```python
from build123d import *

# Parameters (mm, degrees)
SKETCH_W     = 50
SKETCH_H     = 50
PAD_DEPTH    = 3
SKETCH001_R  = 1.05
POCKET_DEPTH = 3.001
CHAMFER_SIZE = 1


with BuildPart() as part:
    # Sketch → Pad (new body)
    with BuildSketch(Plane.XY):
        Rectangle(SKETCH_W, SKETCH_H)
    extrude(amount=PAD_DEPTH)

    # Sketch001 (on Face6 of Pad) → Pocket (cut, through all)
    with BuildSketch(Plane.XY.offset(3)):
        with Locations((-17, 17)):
            Circle(SKETCH001_R)
        with Locations((17, 17)):
            Circle(SKETCH001_R)
        with Locations((17, -17)):
            Circle(SKETCH001_R)
        with Locations((-17, -17)):
            Circle(SKETCH001_R)
    extrude(amount=-POCKET_DEPTH, mode=Mode.SUBTRACT)

    # Chamfer
    chamfer_edges = [part.edges().sort_by_distance(p)[0] for p in [
        (-18.05, 17, 3),
        (15.95, 17, 3),
        (15.95, -17, 3),
        (-18.05, -17, 3),
    ]]
    chamfer(chamfer_edges, length=CHAMFER_SIZE)


solid = part.part
```
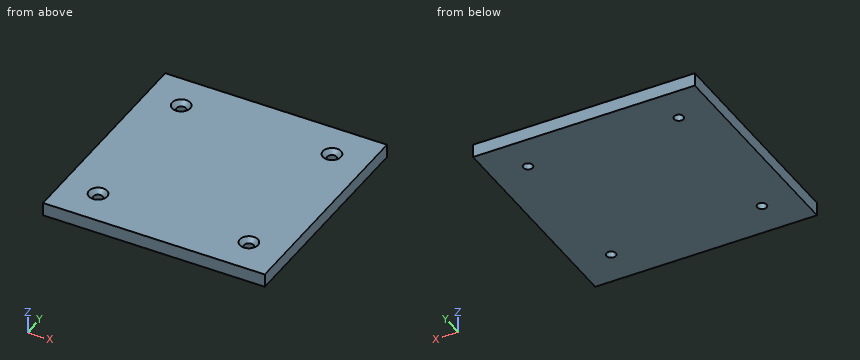
Input: part model. Units: mm. Frame: model coordinates. Coordinates: 2 decimals unless noted, no trailing zeros. Loops run counter-clockwise (first coordinate to the right, second up) from the corner with the lowest first, then second, coordinate; pieces in that order, holes last. Notation, with made-up numbers: M 68.25,3.5 L 82.25,3.5 A24 cw 82.25,20.5 Z; hole C -9,13 d5. An arc over 180 degrees is marked long. One line per item, written item: value.
(1) Line query: line 1 along Y through (x, z) = (17, 0.65); line 2 along X through (y, z) = (-17.5, 0.2). Output: solid intervals per line, ascending. Write a range as from..to.
Filled in:
line 1: -25..-18.05, -15.95..15.95, 18.05..25
line 2: -25..-17.92, -16.08..16.08, 17.92..25
(2) Section A-A (y = 17). Output: boundary loops of the cut face in (x, z), and give its area (3 significant figures).
Filled in:
outline: M -25,0 L -18.05,0 L -18.05,2 L -19.05,3 L -25,3 Z; M -15.95,0 L 15.95,0 L 15.95,2 L 14.95,3 L -14.95,3 L -15.95,2 Z; M 18.05,0 L 25,0 L 25,3 L 19.05,3 L 18.05,2 Z
area: 135 mm^2
(3) Pin query (flat end, axial travel): pin 1 (2.5 mm diameter, centred on x = 17, y = -17, fed in from +Z); pin 2 (3.5 mm diameter, centred on x = -17, y = 17, fed in from +Z). Return the tip coordinate at first contact, or that it passes through.
Filled in:
pin 1: z = 2.2
pin 2: z = 2.7
